from build123d import *

# Parameters (mm, degrees)
F0_W     = 60
F0_H     = 60
F1_DEPTH = 25
F2_R     = 50
F3_T     = -2.5


with BuildPart() as f1:
    # F0 (on Right) → F1 (new body)
    with BuildSketch(Plane.YZ):
        with Locations((30, 4.027068)):
            Rectangle(F0_W, F0_H)
    extrude(amount=F1_DEPTH)

    # F2
    f2_edges = [f1.edges().sort_by_distance(p)[0] for p in [
        (12.5, 60, 34.027068),
    ]]
    fillet(f2_edges, radius=F2_R)

    # F3
    f3_openings = [f1.faces().sort_by_distance(p)[0] for p in [
        (25, 26.702054, 0.729122),
    ]]
    offset(amount=F3_T, openings=f3_openings)


solid = f1.part
Check sheet for the modelled part. Datum: model origin and axes. Units: mm. A direction names the side the tool comes from. Coordinates: 2 decimals unless noted, no trailing zeros. Loops run counter-clockwise (first coordinate to the right, second up) from the corner with the lowest first, then second, coordinate; pieces in that order, holes last. Notation, with made-up numbers: (2.25, 87) -> (17.25, 87) arc R27 ccw to (17.25, 115) -> close; hole circle Ø11 at (70.5, -17.75). An arc over 180 degrees is marked (long way). Answer in a Markdown table with one row per item.
1. Access from +Z, -Z, +X, -X, +Y, -Y to the whole of each face (thin tool, end or side, straight path). Record for faces 4 (the face through (2.5, 30, 4)), 5 (the face through (0, 30, 4)).
Check values:
| item | result |
|---|---|
| face 4 | +X |
| face 5 | +Z, -Z, -X, +Y, -Y |
2. Sectioned sample at C-C, the plane y = 5. Record the boundary of the cut face in (x, z), then the cut area to 4 significant figures.
Check values:
| item | result |
|---|---|
| outline | (0, -25.97) -> (25, -25.97) -> (25, -23.47) -> (2.5, -23.47) -> (2.5, 31.53) -> (25, 31.53) -> (25, 34.03) -> (0, 34.03) -> close |
| area | 262.5 mm2 |
3. Release check for a two-part mould opening along Z. For faces 1 (the face through (12.675, 45.742, 18.992)), 2 (the face through (13.908, 43.955, 17.243)), 3 (the face through (12, 60, -21)) record: released by +Z, released by -Z, zero draft, split by the parting line, or undercut.
Check values:
| item | result |
|---|---|
| face 1 | released by +Z |
| face 2 | undercut |
| face 3 | zero draft |
4. Sectioned sample at B-B, the plane z = -18. Record the boundary of the cut face in (x, y).
Check values:
| item | result |
|---|---|
| outline | (0, 0) -> (25, 0) -> (25, 2.5) -> (2.5, 2.5) -> (2.5, 57.5) -> (25, 57.5) -> (25, 60) -> (0, 60) -> close |
5. Material ranges on line 1 along Y through (x, z) = (20.5, -17); line 2 along Z through (x, y) = (14.75, 5); line 3 along X through (y, z) = (20.5, -14), recorded low to high. Write a range as [from, to].
Check values:
| item | result |
|---|---|
| line 1 | y = [0, 2.5], [57.5, 60] |
| line 2 | z = [-25.97, -23.47], [31.53, 34.03] |
| line 3 | x = [0, 2.5] |
6. Go/stop test with flat-tipped pins: pin 1 (2 mm diameter, centred on x = 16.5, z = 6.5, fed in from +Y); pin 2 (4 mm diameter, centred on x = 8, y = 13.5, fed in from +Z); pin 3 (11 mm diameter, centred on x = 19, y = 24.5, fed in from +Z). Record where each tip stops, or that it passes through.
Check values:
| item | result |
|---|---|
| pin 1 | stops at y = 55.15 |
| pin 2 | stops at z = 34 |
| pin 3 | stops at z = 33.21 |
7. Sectioned sample at A-A, the plane x = 11.25. Record the boundary of the cut face in (y, z).
Check values:
| item | result |
|---|---|
| outline | (0, -25.97) -> (60, -25.97) -> (60, -15.97) arc R50 ccw to (10, 34.03) -> (0, 34.03) -> close; hole (2.5, -23.47) -> (57.5, -23.47) -> (57.5, -15.97) arc R47.5 ccw to (10, 31.53) -> (2.5, 31.53) -> close |
